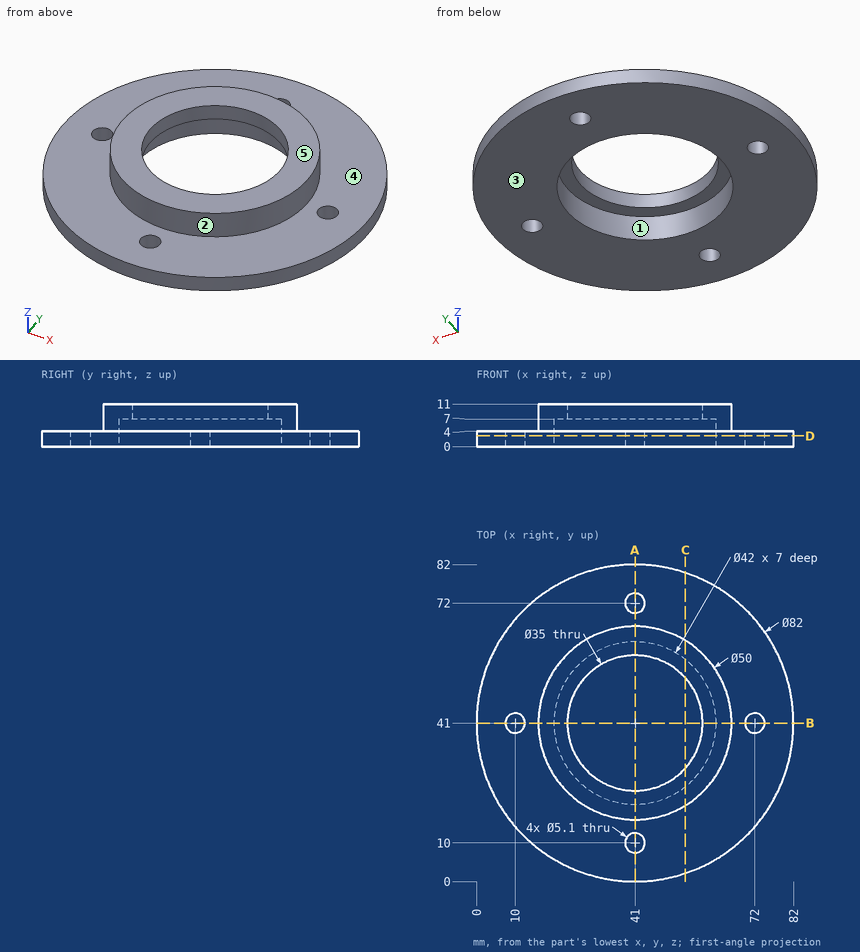
Geometry check sheet. Reference: drawing and pictorial views, mm from the part's lowest x, y, z. A direction names the side the tool comes from. Round coordinates to 2 decimals unless told otherwise and drop trailing zeros. Loops run counter-clockwise (first coordinate to the right, second up) from the corner with the lowest first, then second, coordinate; pieces in that order, holes last. Notation, with made-up numbers: (-6.75, 25.5) - (43.25, 25.5) arc R13 ccw to (43.25, 33.5) - close; hole circle Ø5 at (30, -12). An arc over 180 degrees is marked (long way). One line per question, with ' | ' between items. Start each with the question number.
1. Depth check by flat-ended pin: pin 1 (3 mm diameter, centred on x = 41, y = 10, fed in from -Z); pin 2 (1.5 mm diameter, centred on y = 57, z = 1.5, fed in from -X); pin 3 (1 mm diameter, centred on x = 45, z = 5, fed in from -Y); pin 4 (5 mm diameter, centred on y = 59, z = 2.5, fed in from +X). Enter the tip coordinate at first touch or a pass-through.
2. Tool access check on the marked faces 4 and 5. Record the directions out of +Z, -Z, +X, -X, +Y, -Y that give a thin tool (end or side, any length) a straight path to the whole face; none if there is none.
3. Cross-section at A-A on x = 41. Record the cut outline in (y, z).
4. Cross-section at C-C on x = 54. Record the cut outline in (y, z).
5. Cross-section at D-D on z = 2.75. Record the cut outline in (x, y).
6. Draft check along Y on the marked faces 1, 2 and 3. Enter one of: released by +Y, released by -Y, zero draft, split by the parting line, or undercut.
7. Scan lines: line 1 (Y direction, x = 41, z = 3.5); line 2 (Z direction, x = 78, y = 50); line 3 (Y direction, x = 54.5, z = 3). Record each from-to range of solid material in increasing order. Write a range as [from, to].
Taken from the geometry:
1) pin 1: through | pin 2: x = 2.94 | pin 3: y = 16.25 | pin 4: x = 78.96
2) face 4: +Z | face 5: +Z, +X, -X, +Y, -Y
3) outline: (0, 0) - (7.45, 0) - (7.45, 4) - (0, 4) - close; (12.55, 0) - (20, 0) - (20, 7) - (23.5, 7) - (23.5, 11) - (16, 11) - (16, 4) - (12.55, 4) - close; (58.5, 7) - (62, 7) - (62, 0) - (69.45, 0) - (69.45, 4) - (66, 4) - (66, 11) - (58.5, 11) - close; (74.55, 0) - (82, 0) - (82, 4) - (74.55, 4) - close
4) outline: (2.12, 0) - (24.51, 0) - (24.51, 7) - (29.28, 7) - (29.28, 11) - (19.65, 11) - (19.65, 4) - (2.12, 4) - close; (52.72, 7) - (57.49, 7) - (57.49, 0) - (79.88, 0) - (79.88, 4) - (62.35, 4) - (62.35, 11) - (52.72, 11) - close
5) outline: circle Ø82 at (41, 41); hole circle Ø5.1 at (10, 41); hole circle Ø42 at (41, 41); hole circle Ø5.1 at (41, 10); hole circle Ø5.1 at (41, 72); hole circle Ø5.1 at (72, 41)
6) face 1: undercut | face 2: split by the parting line | face 3: zero draft
7) line 1: [0, 7.45], [12.55, 20], [62, 69.45], [74.55, 82] | line 2: [0, 4] | line 3: [2.29, 24.91], [57.09, 79.71]
